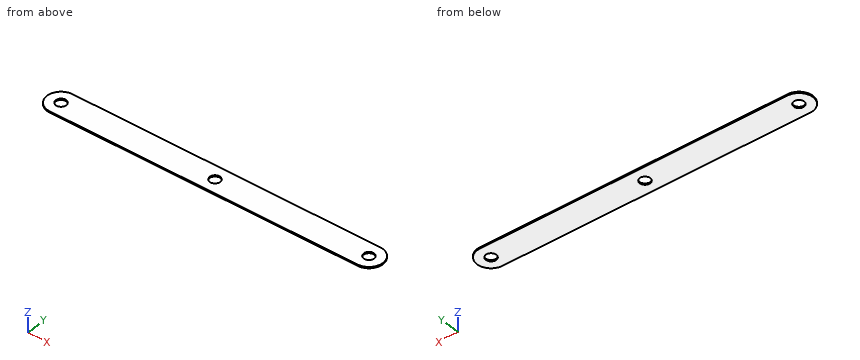
from build123d import *

# Parameters (mm, degrees)
SKETCH1_W           = 279.4
SKETCH1_H           = 25.4
BOSS_EXTRUDE1_DEPTH = 1.2
SKETCH2_R           = 4.7625
CUT_EXTRUDE1_DEPTH  = 2.2
SKETCH3_R           = 4.7625
CUT_EXTRUDE2_DEPTH  = 2.2


with BuildPart() as part:
    # Sketch1 → Boss-Extrude1 (new body)
    with BuildSketch(Plane.XY):
        Rectangle(SKETCH1_W, SKETCH1_H)
        with BuildLine():
            ThreePointArc((139.7, 12.7), (152.4, 0), (139.7, -12.7))
            Line((139.7, -12.7), (139.7, 12.7))
        make_face()
        with BuildLine():
            Line((-139.7, 12.7), (-139.7, -12.7))
            ThreePointArc((-139.7, -12.7), (-152.4, 0), (-139.7, 12.7))
        make_face()
    extrude(amount=BOSS_EXTRUDE1_DEPTH)

    # Sketch2 → Cut-Extrude1 (cut, through all)
    with BuildSketch(Plane.XY.offset(1.2)):
        Circle(SKETCH2_R)
    extrude(amount=-CUT_EXTRUDE1_DEPTH, mode=Mode.SUBTRACT)

    # Sketch3 → Cut-Extrude2 (cut, through all)
    with BuildSketch(Plane.XY.offset(1.2)):
        with Locations((-139.7, 0)):
            Circle(SKETCH3_R)
        with Locations((139.7, 0)):
            Circle(SKETCH3_R)
    extrude(amount=-CUT_EXTRUDE2_DEPTH, mode=Mode.SUBTRACT)


solid = part.part
Read the model definition and answer for the solid it produces. Units are mm, in the model's axes. Give positions to 0.01 mm unless a question says otherwise; leave off trailing zeros. Write each loop counter-clockwise with the first axis right and the second up, starting at its lowest first coordinate (ties: lowest second). Pieces come first, ordered by that corner, then holes. Notation, with made-up numbers: (56, 69) - (74, 69) arc R34 cw to (74, 104) - close; hole circle Ø7 at (49.25, 38). An arc over 180 degrees is marked (long way). Use CSV: the item, a comma, the result in double quotes. Start each with the question number.
Item 1: Consider line 1 (X direction, y = 3.5, z = 0.6); line 2 (Y direction, x = 0, z = 0.4); line 3 (X direction, y = -1, z = 0.55). Determine where each line is inside the solid, lowest interval first.
Item 2: The part is cut by section B-B, the plane y = 0. Give the vertices of the cut face in (x, z), and give its area (3 significant figures).
Item 3: The part is cut by section A-A, the plane x = 0. Give the vertices of the cut face in (y, z).
Item 4: A flat-ended cylindrical pin translates along its axis: P1, Ø7.5, axis at x = 0, y = 0, coming from the +Z side. Find the tip coordinate at first contact, or state that the pin passes through.
Item 5: The part is cut by section C-C, the plane z = 0.4. Give the vertices of the cut face in (x, y) (1 decimal).
Taken from the geometry:
1,line 1,"-151.91 to -142.93, -136.47 to -3.23, 3.23 to 136.47, 142.93 to 151.91"
1,line 2,"-12.7 to -4.76, 4.76 to 12.7"
1,line 3,"-152.36 to -144.36, -135.04 to -4.66, 4.66 to 135.04, 144.36 to 152.36"
2,outline,"(-152.4, 0) - (-144.46, 0) - (-144.46, 1.2) - (-152.4, 1.2) - close; (-134.94, 0) - (-4.76, 0) - (-4.76, 1.2) - (-134.94, 1.2) - close; (4.76, 0) - (134.94, 0) - (134.94, 1.2) - (4.76, 1.2) - close; (144.46, 0) - (152.4, 0) - (152.4, 1.2) - (144.46, 1.2) - close"
2,area,"331 mm2"
3,outline,"(-12.7, 0) - (-4.76, 0) - (-4.76, 1.2) - (-12.7, 1.2) - close; (4.76, 0) - (12.7, 0) - (12.7, 1.2) - (4.76, 1.2) - close"
4,P1,"through"
5,outline,"(-139.7, -12.7) - (139.7, -12.7) arc R12.7 ccw to (139.7, 12.7) - (-139.7, 12.7) arc R12.7 ccw to start; hole circle Ø9.5 at (-139.7, 0); hole circle Ø9.5 at (0, 0); hole circle Ø9.5 at (139.7, 0)"
